For this review, use the dimensioned drawing (mm, ordinates from the lowest corner) and the shaded views. Give positions to 0.01 mm unless a question says otherwise; leave off trailing zeros. Order: outer loops, then holes, each group sorted by start corner. A loop starts at its lowest first (then second) coordinate and runs counter-clockwise, first axis right, second up.
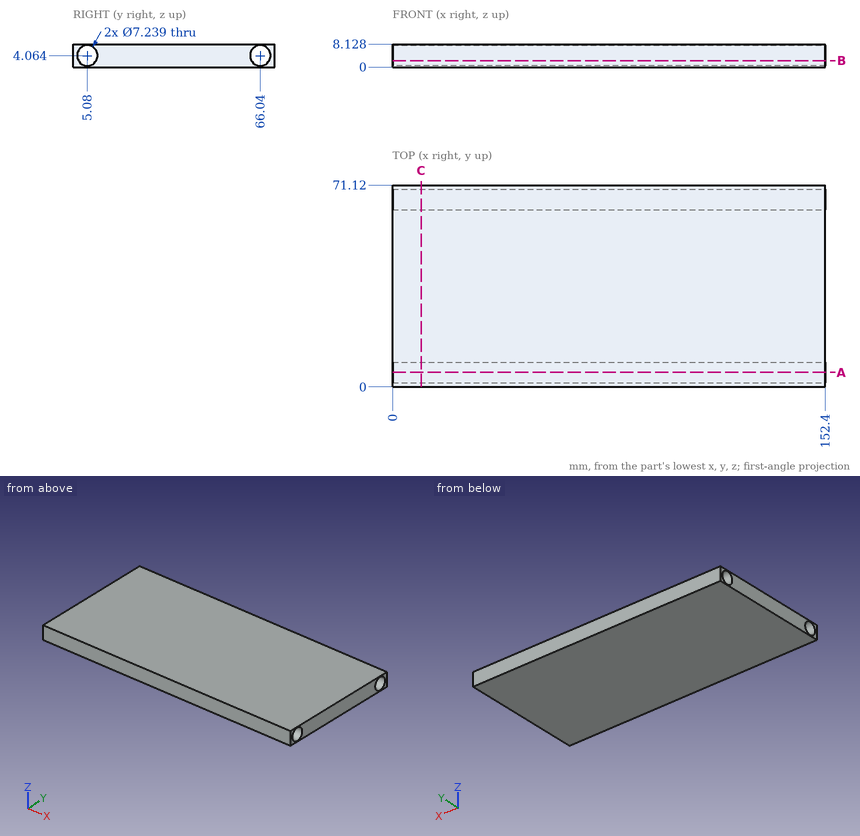
1. Take a section at C-C (x = 10). Write out the cut boundary in (y, z).
2. Take a section at B-B (z = 2.25). Write out the cut boundary in (x, y), and give its area (3 significant figures).
3. To check wall thickness, follow line 1 (Y direction, x = 66, z = 2); line 2 (Y direction, x = 139, z = 1.75); line 3 (Z direction, x = 115, y = 5). State the ranges of each line that lie inside material, in increasing order.
4. Take a section at A-A (y = 5.08). Write out the cut boundary in (x, z).
Answer:
1. outline: (0, 0) - (71.12, 0) - (71.12, 8.13) - (0, 8.13) - close; hole circle Ø7.24 at (5.08, 4.06); hole circle Ø7.24 at (66.04, 4.06)
2. outline: (0, 0) - (152.4, 0) - (152.4, 1.95) - (0, 1.95) - close; (0, 8.21) - (152.4, 8.21) - (152.4, 62.91) - (0, 62.91) - close; (0, 69.17) - (152.4, 69.17) - (152.4, 71.12) - (0, 71.12) - close
2. area: 8,930 mm2
3. line 1: y = 0 to 2.11, 8.05 to 63.07, 69.01 to 71.12
3. line 2: y = 0 to 2.3, 7.86 to 63.26, 68.82 to 71.12
3. line 3: z = 0 to 0.45, 7.68 to 8.13
4. outline: (0, 0) - (152.4, 0) - (152.4, 0.44) - (0, 0.44) - close; (0, 7.68) - (152.4, 7.68) - (152.4, 8.13) - (0, 8.13) - close
